The model under review builds one solid part; all positions refer to its coordinate system, in mm. A direction names the side the tool comes from. Round coordinates to 2 decimals unless told otherwise and drop trailing zeros. Order: outer loops, then holes, each group sorted by start corner. A loop starts at its lowest first (then second) coordinate and runs counter-clockwise, first axis right, second up.
```python
from build123d import *

# Parameters (mm, degrees)
SALIENTE_EXTRUIR1_DEPTH    = 30
CORTAR_EXTRUIR2_DEPTH      = 32
CORTAR_EXTRUIR2_DEPTH_BACK = 9
CROQUIS2_R                 = 10
CORTAR_EXTRUIR3_DEPTH      = 90
CORTAR_EXTRUIR4_DEPTH      = 130.248290693
CORTAR_EXTRUIR5_DEPTH      = 130.248290693
REDONDEO2_R                = 10
REDONDEO3_R                = 10
REDONDEO4_R                = 10


with BuildPart() as part:
    # Croquis1 → Saliente-Extruir1 (new, symmetric)
    with BuildSketch(Plane.XY):
        Polygon((0, 0), (50, 0), (76, 26), (122.086529343, 26), (122.086529343, 30), (74.343145751, 30), (48.343145751, 4), (0, 4), align=None)
    extrude(amount=SALIENTE_EXTRUIR1_DEPTH, both=True)

    # Croquis2 → Cortar-Extruir2 (cut, two sides: drawn at the far end of the back side and taken through both)
    with BuildSketch(Plane(origin=(0, 0, 0), x_dir=(1, 0, 0), z_dir=(0, 1, 0)).offset(-CORTAR_EXTRUIR2_DEPTH_BACK)):
        with Locations(Location((26, 0, 0), (0, 0, 90))):
            Circle(CROQUIS2_R)
    extrude(amount=CORTAR_EXTRUIR2_DEPTH + CORTAR_EXTRUIR2_DEPTH_BACK, mode=Mode.SUBTRACT)

    # Croquis3 → Cortar-Extruir3 (cut)
    with BuildSketch(Plane(origin=(0, 0, 0), x_dir=(1, 0, 0), z_dir=(0, 1, 0))):
        with BuildLine():
            Line((122.086529343, -7), (101.086529343, -7))
            ThreePointArc((101.086529343, -7), (94.086529343, 0), (101.086529343, 7))
            Line((101.086529343, 7), (122.086529343, 7))
            ThreePointArc((122.086529343, 7), (129.086529343, 0), (122.086529343, -7))
        make_face()
    extrude(amount=CORTAR_EXTRUIR3_DEPTH, mode=Mode.SUBTRACT)

    # Croquis4 → Cortar-Extruir4 (cut, through all)
    with BuildSketch(Plane(origin=(0, 0, 0), x_dir=(1, 0, 0), z_dir=(0, 1, 0))):
        Polygon((98.214837547, 30), (122.086529343, 8), (122.086529343, 30), align=None)
    cortar_extruir4 = extrude(amount=CORTAR_EXTRUIR4_DEPTH, mode=Mode.SUBTRACT)

    # Simetría1: Cortar-Extruir4 across plane
    add(cortar_extruir4.mirror(Plane.XY), mode=Mode.SUBTRACT)

    # Croquis5 → Cortar-Extruir5 (cut, through all)
    with BuildSketch(Plane(origin=(0, 0, 0), x_dir=(1, 0, 0), z_dir=(0, 1, 0))):
        with BuildLine():
            Line((0, 30), (24.171572875, 30))
            ThreePointArc((24.171572875, 30), (10.356957759, 25.984893458), (0, 16))
            Line((0, 16), (0, 30))
        make_face()
    cortar_extruir5 = extrude(amount=CORTAR_EXTRUIR5_DEPTH, mode=Mode.SUBTRACT)

    # Simetría2: Cortar-Extruir5 across plane
    add(cortar_extruir5.mirror(Plane.XY), mode=Mode.SUBTRACT)

    # Redondeo2
    redondeo2_edges = [part.edges().sort_by_distance(p)[0] for p in [
        (48.343145751, 4, 0),
    ]]
    fillet(redondeo2_edges, radius=REDONDEO2_R)

    # Redondeo3
    redondeo3_edges = [part.edges().sort_by_distance(p)[0] for p in [
        (74.343145751, 30, 0),
    ]]
    fillet(redondeo3_edges, radius=REDONDEO3_R)

    # Redondeo4
    redondeo4_edges = [part.edges().sort_by_distance(p)[0] for p in [
        (76, 26, 0),
        (50, 0, 0),
    ]]
    fillet(redondeo4_edges, radius=REDONDEO4_R)


solid = part.part
```
(1) Consider section A-A (x = 34). Write out the cut boundary in (y, z).
Data:
outline: (0, -30) - (4, -30) - (4, -6) - (0, -6) - close; (0, 6) - (4, 6) - (4, 30) - (0, 30) - close
(2) For faces 1 (the flat face through (112, 28, 7)), 2 (the flat face through (63, 13, 0)), 3 (the flat face through (17, 4, -6)), list the 3-axis set-ups (+Z, -Z, +X, -X, +Y, -Y) from which the entire face can be reached by the end or side of a thin tool; tool diameter is ignored.
Data:
face 1: +X, +Y, -Y
face 2: +Z, -Z, +X, -Y
face 3: +Z, -Z, -X, +Y
(3) Consider section C-C (z = 14). Write out the cut boundary in (x, y), and give its area (3 significant figures).
Data:
outline: (0, 0) - (45.86, 0) arc R10 ccw to (52.93, 2.93) - (73.07, 23.07) arc R10 cw to (80.14, 26) - (115.58, 26) - (115.58, 30) - (78.49, 30) arc R10 ccw to (71.41, 27.07) - (51.27, 6.93) arc R10 cw to (44.2, 4) - (0, 4) - close
area: 505 mm2
(4) Consider section D-D (x = 95.5). Write out the cut boundary in (y, z), and give its area (3 significant figures).
Data:
outline: (26, -30) - (30, -30) - (30, -4.22) - (26, -4.22) - close; (26, 4.22) - (30, 4.22) - (30, 30) - (26, 30) - close
area: 206 mm2
(5) Insertion check: pin 1 (10 mm diameter, centred on x = 73, z = -4.5, fed in from +Y); pin 2 (2 mm diameter, centred on x = 69.5, z = -23.5, fed in from -Y); pin 3 (13.5 mm diameter, centred on x = 25, z = 13, fed in from +Y). Each pin has a flat end and moves straight along its axis. Give the tip position at first contact, or say it passes through.
Data:
pin 1: stops at y = 29.99
pin 2: stops at y = 18.5
pin 3: stops at y = 4
(6) Draft analysis for pull direction Z (two halves, no side actions). For faces 4 (the cylindrical face through (10.533, 1.972, -26.086)), 5 (the cylindrical face through (94.09, 27.97, 0.15)), 6 (the cylindrical face through (74.61, 29.22, 0.42)), state which applies: pulls with the +Z half, pulls with the -Z half, needs draft (parallel to the pull), parting line crosses it, or undercut.
Data:
face 4: pulls with the -Z half
face 5: undercut
face 6: needs draft
(7) Consider section B-B (z = 0). Write out the cut boundary in (x, y), and give its area (3 significant figures).
Data:
outline: (0, 0) - (16, 0) - (16, 4) - (0, 4) - close; (36, 0) - (45.86, 0) arc R10 ccw to (52.93, 2.93) - (73.07, 23.07) arc R10 cw to (80.14, 26) - (94.09, 26) - (94.09, 30) - (78.49, 30) arc R10 ccw to (71.41, 27.07) - (51.27, 6.93) arc R10 cw to (44.2, 4) - (36, 4) - close
area: 339 mm2
(8) To check wall thickness, follow probe 1 along Y at (x, z) = (44.5, -20.5); probe 2 along X at (y, z) = (2.65, 0); probe 3 along Y at (x, z) = (83, -17.5). State the ranges of each line that lie inside material, in increasing order.
Data:
probe 1: y = 0 to 4
probe 2: x = 0 to 16, 36 to 52.64
probe 3: y = 26 to 30
